Here's how the part is built. I have some questions about the finished solid (model axes, mm). A direction names the side the tool comes from. Round coordinates to 2 decimals unless told otherwise and drop trailing zeros. Loops run counter-clockwise (first coordinate to the right, second up) from the corner with the lowest first, then second, coordinate; pieces in that order, holes last. Notation, with made-up numbers: M 48.5,88.5 L 98.5,88.5 A5 cw 98.5,97.5 Z; hole C -26,88.25 d1. An arc over 180 degrees is marked long. Answer as a JSON object with one key per item and string values.
from build123d import *

# Parameters (mm, degrees)
SKETCH_1_R          = 25
SKETCH_1_R_2        = 15
EXTRUDE_1_DEPTH     = 32
EXTRUDE_START       = -32
SKETCH_2_W          = 60.925429914
SKETCH_2_H          = 40
EXTRUDE_2_DEPTH     = 25
CUT_EXTRUDE_1_DEPTH = 10
SKETCH_4_R          = 5
CUT_EXTRUDE_2_DEPTH = 48
CUT_EXTRUDE_START   = -48
CUT_EXTRUDE_3_DEPTH = 48


with BuildPart() as part:
    # 草图1 → 凸台-拉伸1 (new body)
    with BuildSketch(Plane(origin=(0, 0, 0), x_dir=(1, 0, 0), z_dir=(0, 1, 0))):
        with Locations(Location((0, 0, 0), (0, 0, 270))):
            Circle(SKETCH_1_R)
        with Locations(Location((0, 0, 0), (0, 0, 270))):
            Circle(SKETCH_1_R_2, mode=Mode.SUBTRACT)
    extrude(amount=EXTRUDE_1_DEPTH)

    # 草图2 → 凸台-拉伸2 (add)
    with BuildSketch(Plane(origin=(0, 32, 0), x_dir=(1, 0, 0), z_dir=(0, 1, 0)).offset(EXTRUDE_START)):
        with Locations((45.537285043, 0)):
            Rectangle(SKETCH_2_W, SKETCH_2_H)
    extrude(amount=EXTRUDE_2_DEPTH)

    # 草图3 → 切除-拉伸1 (cut)
    with BuildSketch(Plane(origin=(0, 25, 0), x_dir=(1, 0, 0), z_dir=(0, 1, 0))):
        with BuildLine():
            Line((76, 14), (33.94427191, 14))
            ThreePointArc((33.94427191, 14), (28.467046335, 10.449489743), (29.472135955, 4))
            ThreePointArc((29.472135955, 4), (31, 0), (29.472135955, -4))
            ThreePointArc((29.472135955, -4), (28.467046335, -10.449489743), (33.94427191, -14))
            Line((33.94427191, -14), (76, -14))
            Line((76, -14), (76, 14))
        make_face()
    extrude(amount=-CUT_EXTRUDE_1_DEPTH, mode=Mode.SUBTRACT)

    # 草图4 → 切除-拉伸2 (cut)
    with BuildSketch(Plane(origin=(0, 15, 0), x_dir=(1, 0, 0), z_dir=(0, 1, 0))):
        with Locations(Location((46, 0, 0), (0, 0, 270))):
            Circle(SKETCH_4_R)
        with Locations(Location((64, 0, 0), (0, 0, 270))):
            Circle(SKETCH_4_R)
    extrude(amount=-CUT_EXTRUDE_2_DEPTH, mode=Mode.SUBTRACT)

    # 草图5 → 切除-拉伸3 (cut)
    with BuildSketch(Plane(origin=(0, 32, 0), x_dir=(1, 0, 0), z_dir=(0, 1, 0)).offset(CUT_EXTRUDE_START)):
        with BuildLine():
            Line((-20, 4), (-14.456832295, 4))
            ThreePointArc((-14.456832295, 4), (-15, 0), (-14.456832295, -4))
            Line((-14.456832295, -4), (-20, -4))
            Line((-20, -4), (-20, 4))
        make_face()
    extrude(amount=CUT_EXTRUDE_3_DEPTH, mode=Mode.SUBTRACT)


solid = part.part
Item 1: I'm going to push flat-ended pins straight in: pin 1 Ø4 at (x, y) = (37, 16) entering from +Z; pin 2 Ø14 at (x, z) = (54.5, -1.5) entering from +Y; pin 3 Ø5 at (y, z) = (24.5, 5) entering from -X; pin 4 Ø6 at (x, z) = (46, 0) entering from -Y. Where does each tip first touch, or does it pass through?
Resolved:
{"pin 1": "z = 20", "pin 2": "y = 15", "pin 3": "x = -24.87", "pin 4": "through"}
Item 2: If we mould it in two halves opening along Z, with no side actions, what happens to faces 6 (the face through (45, 12, 20)), 7 (the face through (52, 15, 0)), 8 (the face through (-11, 32, 11))? For each: pulls with the +Z half, pulls with the -Z half, needs draft (parallel to the pull), parting line crosses it, or undercut.
Resolved:
{"face 6": "pulls with the +Z half", "face 7": "undercut", "face 8": "needs draft"}
Item 3: I want a section at D-D, the plane z = -12.5. Please give me the cut outline in (x, y).
Resolved:
{"outline": "M -21.65,0 L -8.29,0 L -8.29,32 L -21.65,32 Z; M 8.29,0 L 76,0 L 76,15 L 29.98,15 L 29.98,25 L 21.65,25 L 21.65,32 L 8.29,32 Z"}
Item 4: On a 3-axis mill with a long thin cutter (end or side, diameter ignored), from which of +Z, -Z, +X, -X, +Y, -Y can I reach the whole of each face in a straight line? I mean faces 1 (the face through (25, 0, 0)), 2 (the face through (76, 10, 0)), 3 (the face through (55, 20, 14)), 4 (the face through (-20, 16, 0)), 5 (the face through (45, 12, -20)). Say none if no direction works.
Resolved:
{"face 1": "+Z, -Z, +X, -X, -Y", "face 2": "+Z, -Z, +X, +Y, -Y", "face 3": "+X, +Y", "face 4": "+Y, -Y", "face 5": "-Z, +X, +Y, -Y"}
Item 5: I want a section at B-B, the plane y = 23. Please give me the cut outline in (x, z), then the cut area to 3 significant figures.
Resolved:
{"outline": "M 15.07,-20 L 76,-20 L 76,-14 L 33.94,-14 A6 cw 29.47,-4 A6 ccw 29.47,4 A6 cw 33.94,14 L 76,14 L 76,20 L 15.07,20 L 15.07,19.94 A25 ccw long 15.07,-19.94 Z; hole M -20,-4 L -14.46,-4 A15 ccw long -14.46,4 L -20,4 Z", "area": "2,070 mm²"}
Item 6: I want a section at C-C, the plane x = 64. Please give me the cut outline in (y, z).
Resolved:
{"outline": "M 0,-20 L 25,-20 L 25,-14 L 15,-14 L 15,-5 L 0,-5 Z; M 0,5 L 15,5 L 15,14 L 25,14 L 25,20 L 0,20 Z"}
Item 7: I want a section at A-A, the plane z = 0. Please give me the cut outline in (x, y).
Resolved:
{"outline": "M -25,0 L -20,0 L -20,32 L -25,32 Z; M 15,0 L 41,0 L 41,15 L 31,15 L 31,25 L 25,25 L 25,32 L 15,32 Z; M 51,0 L 59,0 L 59,15 L 51,15 Z; M 69,0 L 76,0 L 76,15 L 69,15 Z"}
Item 8: Please list where these lines run through material, in increasing order: probe 1 along X at (y, z) = (13, 0); probe 2 along Z at (x, y) = (0, 6); probe 3 along Z at (x, y) = (36, 21.5). Write a range as from..to.
Resolved:
{"probe 1": "-25..-20, 15..41, 51..59, 69..76", "probe 2": "-25..-15, 15..25", "probe 3": "-20..-14, 14..20"}
